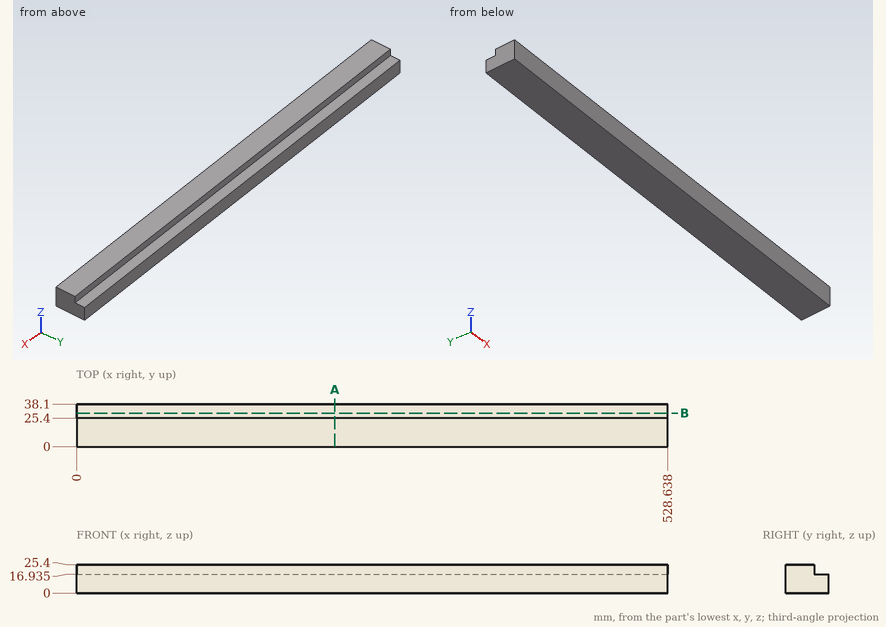
For this review, use the dimensioned drawing (mm, ordinates from the lowest corner) and the shaded views. Give positions to 0.01 mm unless a question says otherwise; leave off trailing zeros. Write each loop counter-clockwise with the first axis right and the second up, starting at its lowest first coordinate (ties: lowest second). Pieces come first, ordered by that corner, then holes.
(1) Consider section B-B, the plane y = 30. Give the boundary of the cut face in (x, z) (1 decimal), and give its area (3 significant figures).
(2) For P1, Ø9.5, axis at x = 356, z = 19.5, coming from the +Y side; P2, Ø1, axis at x = 247.5, y = 31, coming from the +Z side (1 decimal), all flat-tipped, find the tip position at first contact; note any pin that passes through.
(3) To check wall thickness, follow L1, parallel to Z at x = 376, y = 34.5 (1 decimal); L2, parallel to Y at x = 371.5, z = 18.75. State the ranges of each line that lie inside material, in increasing order.
(4) Consider section A-A, the plane x = 231. Give the boundary of the cut face in (y, z) (1 decimal).
Returned:
1. outline: (0, 0) - (528.6, 0) - (528.6, 16.9) - (0, 16.9) - close
1. area: 8,950 mm2
2. P1: stops at y = 38.1
2. P2: stops at z = 16.9
3. L1: z = 0 to 16.9
3. L2: y = 0 to 25.4
4. outline: (0, 0) - (38.1, 0) - (38.1, 16.9) - (25.4, 16.9) - (25.4, 25.4) - (0, 25.4) - close
